from build123d import *

# Parameters (mm, degrees)
SKETCH_1_R      = 2.5
EXTRUDE_1_DEPTH = 100


with BuildPart() as part:
    # 草图1 → 凸台-拉伸1 (new body)
    with BuildSketch(Plane.XY):
        with BuildLine():
            Line((2.839339828, 3.9), (5.5, 6.560660172))
            Line((5.5, 6.560660172), (5.5, 8.2))
            Line((5.5, 8.2), (3.1, 8.2))
            Line((3.1, 8.2), (3.1, 8.965473865))
            ThreePointArc((3.1, 8.965473865), (3.158578644, 9.106895221), (3.3, 9.165473865))
            Line((3.3, 9.165473865), (3.589843476, 9.165473865))
            Line((3.589843476, 9.165473865), (3.589843476, 9.8))
            ThreePointArc((3.589843476, 9.8), (3.64842212, 9.941421356), (3.789843476, 10))
            Line((3.789843476, 10), (8.5, 10))
            ThreePointArc((8.5, 10), (9.560660172, 9.560660172), (10, 8.5))
            Line((10, 8.5), (10, 3.789843476))
            ThreePointArc((10, 3.789843476), (9.941421356, 3.64842212), (9.8, 3.589843476))
            Line((9.8, 3.589843476), (9.165473865, 3.589843476))
            Line((9.165473865, 3.589843476), (9.165473865, 3.3))
            ThreePointArc((9.165473865, 3.3), (9.106895221, 3.158578644), (8.965473865, 3.1))
            Line((8.965473865, 3.1), (8.2, 3.1))
            Line((8.2, 3.1), (8.2, 5.5))
            Line((8.2, 5.5), (6.560660172, 5.5))
            Line((6.560660172, 5.5), (3.9, 2.839339828))
            Line((3.9, 2.839339828), (3.9, -2.839339828))
            Line((3.9, -2.839339828), (6.560660172, -5.5))
            Line((6.560660172, -5.5), (8.2, -5.5))
            Line((8.2, -5.5), (8.2, -3.1))
            Line((8.2, -3.1), (8.965473865, -3.1))
            ThreePointArc((8.965473865, -3.1), (9.106895221, -3.158578644), (9.165473865, -3.3))
            Line((9.165473865, -3.3), (9.165473865, -3.589843476))
            Line((9.165473865, -3.589843476), (9.8, -3.589843476))
            ThreePointArc((9.8, -3.589843476), (9.941421356, -3.64842212), (10, -3.789843476))
            Line((10, -3.789843476), (10, -8.5))
            ThreePointArc((10, -8.5), (9.560660172, -9.560660172), (8.5, -10))
            Line((8.5, -10), (3.789843476, -10))
            ThreePointArc((3.789843476, -10), (3.64842212, -9.941421356), (3.589843476, -9.8))
            Line((3.589843476, -9.8), (3.589843476, -9.165473865))
            Line((3.589843476, -9.165473865), (3.3, -9.165473865))
            ThreePointArc((3.3, -9.165473865), (3.158578644, -9.106895221), (3.1, -8.965473865))
            Line((3.1, -8.965473865), (3.1, -8.2))
            Line((3.1, -8.2), (5.5, -8.2))
            Line((5.5, -8.2), (5.5, -6.560660172))
            Line((5.5, -6.560660172), (2.839339828, -3.9))
            Line((2.839339828, -3.9), (-2.839339828, -3.9))
            Line((-2.839339828, -3.9), (-5.5, -6.560660172))
            Line((-5.5, -6.560660172), (-5.5, -8.2))
            Line((-5.5, -8.2), (-3.1, -8.2))
            Line((-3.1, -8.2), (-3.1, -8.965473865))
            ThreePointArc((-3.1, -8.965473865), (-3.158578644, -9.106895221), (-3.3, -9.165473865))
            Line((-3.3, -9.165473865), (-3.589843476, -9.165473865))
            Line((-3.589843476, -9.165473865), (-3.589843476, -9.8))
            ThreePointArc((-3.589843476, -9.8), (-3.64842212, -9.941421356), (-3.789843476, -10))
            Line((-3.789843476, -10), (-8.5, -10))
            ThreePointArc((-8.5, -10), (-9.560660172, -9.560660172), (-10, -8.5))
            Line((-10, -8.5), (-10, -3.789843476))
            ThreePointArc((-10, -3.789843476), (-9.941421356, -3.64842212), (-9.8, -3.589843476))
            Line((-9.8, -3.589843476), (-9.165473865, -3.589843476))
            Line((-9.165473865, -3.589843476), (-9.165473865, -3.3))
            ThreePointArc((-9.165473865, -3.3), (-9.106895221, -3.158578644), (-8.965473865, -3.1))
            Line((-8.965473865, -3.1), (-8.2, -3.1))
            Line((-8.2, -3.1), (-8.2, -5.5))
            Line((-8.2, -5.5), (-6.560660172, -5.5))
            Line((-6.560660172, -5.5), (-3.9, -2.839339828))
            Line((-3.9, -2.839339828), (-3.9, 2.839339828))
            Line((-3.9, 2.839339828), (-6.560660172, 5.5))
            Line((-6.560660172, 5.5), (-8.2, 5.5))
            Line((-8.2, 5.5), (-8.2, 3.1))
            Line((-8.2, 3.1), (-8.965473865, 3.1))
            ThreePointArc((-8.965473865, 3.1), (-9.106895221, 3.158578644), (-9.165473865, 3.3))
            Line((-9.165473865, 3.3), (-9.165473865, 3.589843476))
            Line((-9.165473865, 3.589843476), (-9.8, 3.589843476))
            ThreePointArc((-9.8, 3.589843476), (-9.941421356, 3.64842212), (-10, 3.789843476))
            Line((-10, 3.789843476), (-10, 8.5))
            ThreePointArc((-10, 8.5), (-9.560660172, 9.560660172), (-8.5, 10))
            Line((-8.5, 10), (-3.789843476, 10))
            ThreePointArc((-3.789843476, 10), (-3.64842212, 9.941421356), (-3.589843476, 9.8))
            Line((-3.589843476, 9.8), (-3.589843476, 9.165473865))
            Line((-3.589843476, 9.165473865), (-3.3, 9.165473865))
            ThreePointArc((-3.3, 9.165473865), (-3.158578644, 9.106895221), (-3.1, 8.965473865))
            Line((-3.1, 8.965473865), (-3.1, 8.2))
            Line((-3.1, 8.2), (-5.5, 8.2))
            Line((-5.5, 8.2), (-5.5, 6.560660172))
            Line((-5.5, 6.560660172), (-2.839339828, 3.9))
            Line((-2.839339828, 3.9), (2.839339828, 3.9))
        make_face()
        Circle(SKETCH_1_R, mode=Mode.SUBTRACT)
    extrude(amount=EXTRUDE_1_DEPTH)


solid = part.part
Model file for the job. Use its own axes, mm. A direction names the side the tool comes from. Give positions to 0.01 mm unless a question says otherwise; leave off trailing zeros. Loops run counter-clockwise (first coordinate to the right, second up) from the corner with the lowest first, then second, coordinate; pieces in that order, holes last.
1) Pull direction X, two halves, no side cores. Call faces 1 (the flat face through (-5.25, -4.19, 49.3)), 2 (the flat face through (2, 2, 0)), 3 (the flat face through (-10, -6, 49)), 4 (the flat face through (3.9, 0, 49)): +X half, -X half, draft (parallel to the pull), parting line (faces both ways), or undercut.
2) Saw through at A-A (x = 0). Write the cut outline in (y, z).
3) Wall check: line 1 (Y direction, x = 0, z = 62); line 2 (Y direction, x = -7, z = 8.5). Give the ranges that are in metal, low to high.
4) Tool access for faces 5 (the flat face through (4, 8.2, 49)), 6 (the flat face through (0, 3.9, 49)), 7 (the flat face through (10, -6, 49)): list every direction of +Z, -Z, +X, -X, +Y, -Y with a clear straight run to the whole face (end or side of a thin tool).
5) Flat gauge pins, fed straight in: pin 1 Ø12 at (x, y) = (1.5, 1.5) entering from +Z; pin 2 Ø3 at (y, z) = (-0.5, 67) entering from +X; pin 3 Ø1.7 at (y, z) = (1, 32) entering from -X. Where does each tip first touch, or does it go through?
Answer block:
1. face 1: undercut
1. face 2: draft
1. face 3: -X half
1. face 4: +X half
2. outline: (-3.9, 0) - (-2.5, 0) - (-2.5, 100) - (-3.9, 100) - close; (2.5, 0) - (3.9, 0) - (3.9, 100) - (2.5, 100) - close
3. line 1: y = -3.9 to -2.5, 2.5 to 3.9
3. line 2: y = -10 to -5.5, 5.5 to 10
4. face 5: +Z, -Z
4. face 6: +Z, -Z, +Y
4. face 7: +Z, -Z, +X, +Y, -Y
5. pin 1: stops at z = 100
5. pin 2: stops at x = 3.9
5. pin 3: stops at x = -3.9
